from build123d import *

# Parameters (mm, degrees)
CROQUIS1_R               = 1.55
CROQUIS1_R_2             = 4
SALIENTE_EXTRUIR10_DEPTH = 3
CROQUIS2_R               = 8
CROQUIS2_R_2             = 1.55
CORTAR_EXTRUIR1_DEPTH    = 3
CROQUIS3_OUTSIDE_W       = 98.706
CROQUIS3_OUTSIDE_H       = 99.406
CROQUIS3_OUTSIDE_R       = 4
CROQUIS3_OUTSIDE_R_2     = 8
CROQUIS3_OUTSIDE_R_3     = 1.55
CORTAR_EXTRUIR2_DEPTH    = 3
REDONDEO1_R              = 6
REDONDEO2_R              = 3


with BuildPart() as part:
    # Croquis1 → Saliente-Extruir10 (new body)
    with BuildSketch(Plane(origin=(0, 0, 0), x_dir=(1, 0, 0), z_dir=(0, 1, 0))):
        Polygon((0, 0), (0, 38.7), (10, 38.7), (10, 42), (0, 42), (0, 72), (69.3, 72), (75.3, 72), (75.3, 52), (75.3, 42), (69.3, 42), (69.3, 51.7), (66, 51.7), (66, 42), (50, 42), (50, 38.7), (69.3, 38.7), (69.3, 0), (69.3, -4), (0, -4), align=None)
        with Locations((30, 40.2)):
            Circle(CROQUIS1_R, mode=Mode.SUBTRACT)
        with Locations((67.8, 61.7)):
            Circle(CROQUIS1_R, mode=Mode.SUBTRACT)
        with Locations((12.5, 9.4)):
            Circle(CROQUIS1_R_2, mode=Mode.SUBTRACT)
    extrude(amount=SALIENTE_EXTRUIR10_DEPTH)

    # Croquis2 → Cortar-Extruir1 (cut)
    with BuildSketch(Plane(origin=(0, 3, 0), x_dir=(1, 0, 0), z_dir=(0, 1, 0))):
        with Locations((29.5, 9.7)):
            Circle(CROQUIS2_R)
        with Locations((12.5, 17.4)):
            Circle(CROQUIS2_R_2)
        with Locations((12.5, 1.4)):
            Circle(CROQUIS2_R_2)
    extrude(amount=-CORTAR_EXTRUIR1_DEPTH, mode=Mode.SUBTRACT)

    # Croquis3 outside → Cortar-Extruir2 (cut)
    with BuildSketch(Plane(origin=(0, 3, 0), x_dir=(1, 0, 0), z_dir=(0, 1, 0))):
        with Locations((37.65, 34)):
            Rectangle(CROQUIS3_OUTSIDE_W, CROQUIS3_OUTSIDE_H)
        with BuildLine():
            Line((75.3, 72), (63, 72))
            ThreePointArc((63, 72), (34.270978976, 52.034382388), (0, 45))
            Line((0, 45), (0, 42))
            Line((0, 42), (10, 42))
            Line((10, 42), (10, 38.7))
            Line((10, 38.7), (0, 38.7))
            Line((0, 38.7), (0, 9.7))
            ThreePointArc((0, 9.7), (5.916961411, -0.92608126), (18.066176471, -1.492304477))
            ThreePointArc((18.066176471, -1.492304477), (19.571107199, -2.84659666), (21.235013612, -4))
            Line((21.235013612, -4), (37.764986388, -4))
            ThreePointArc((37.764986388, -4), (43.432691452, 1.833608903), (45.5, 9.7))
            ThreePointArc((45.5, 9.7), (54.274410069, 25.678480622), (69.3, 36))
            Line((69.3, 36), (69.3, 38.7))
            Line((69.3, 38.7), (50, 38.7))
            Line((50, 38.7), (50, 42))
            Line((50, 42), (66, 42))
            Line((66, 42), (66, 51.7))
            Line((66, 51.7), (69.3, 51.7))
            Line((69.3, 51.7), (69.3, 42))
            Line((69.3, 42), (75.3, 42))
            Line((75.3, 42), (75.3, 72))
        make_face(mode=Mode.SUBTRACT)
        with Locations((12.5, 9.4)):
            Circle(CROQUIS3_OUTSIDE_R)
        with Locations((29.5, 9.7)):
            Circle(CROQUIS3_OUTSIDE_R_2)
        with Locations((30, 40.2)):
            Circle(CROQUIS3_OUTSIDE_R_3)
        with Locations((67.8, 61.7)):
            Circle(CROQUIS3_OUTSIDE_R_3)
    extrude(amount=-CORTAR_EXTRUIR2_DEPTH, mode=Mode.SUBTRACT)

    # Redondeo1
    redondeo1_edges = [part.edges().sort_by_distance(p)[0] for p in [
        (75.3, 1.5, -72),
    ]]
    fillet(redondeo1_edges, radius=REDONDEO1_R)

    # Redondeo2
    redondeo2_edges = [part.edges().sort_by_distance(p)[0] for p in [
        (0, 1.5, -45),
    ]]
    fillet(redondeo2_edges, radius=REDONDEO2_R)


solid = part.part
Source: CAD feature listing. Evaluate the final solid. Frame: model axes, mm. A direction names the side the tool comes from. Give positions to 0.01 mm unless a question says otherwise; leave off trailing zeros. Order: outer loops, then holes, each group sorted by start corner. A loop starts at its lowest first (then second) coordinate and runs counter-clockwise, first axis right, second up. Notation, with made-up numbers: (59, 86) -> (112, 86) arc R28 cw to (112, 119) -> close; hole circle Ø4 at (-3.75, 50). An arc over 180 degrees is marked (long way). Write item = value, one per line.
Item 1: Section query B-B (x = 29.5). Output: boundary loops of the cut face in (y, z), then the cut area to 3 significant figures.
Check result:
outline = (0, -50.15) -> (3, -50.15) -> (3, -41.67) -> (0, -41.67) -> close; (0, -38.73) -> (3, -38.73) -> (3, -17.7) -> (0, -17.7) -> close; (0, -1.7) -> (3, -1.7) -> (3, 4) -> (0, 4) -> close
area = 106 mm²
Item 2: Section query C-C (x = 15.5). Output: boundary loops of the cut face in (y, z), then the cut area to 3 significant figures.
Check result:
outline = (0, -46.39) -> (3, -46.39) -> (3, -12.05) -> (0, -12.05) -> close; (0, -6.75) -> (3, -6.75) -> (3, 2.43) -> (0, 2.43) -> close
area = 131 mm²
Item 3: Contact query for flat-ended pins moving along their axis: pin 1 (0.9 mm diameter, centred on x = 61.5, y = 2, fed in from +Z); pin 2 (1.5 mm diameter, centred on x = 40, y = 0.5, fed in from -Z); pin 3 (1.5 mm diameter, centred on y = 1, z = -40, fed in from +X). Output: stop coordinate, or through.
Check result:
pin_1 = -31.63
pin_2 = -55.13
pin_3 = 50
Item 4: Section query A-A (y = 1.2). State how many separate pieces and enclosed holes the cut face has, then the cut area to 3 significant figures.
Check result:
separate_pieces = 1
enclosed_holes = 6
area = 3,020 mm²
Item 5: Mould query, pull axis Z, two halves, no side actions, for faces 1 (the face through (19.55, 1.52, 2.83)), 2 (the face through (75.3, 1, -54)), 3 (the face through (60, 1, -38.7)). Classes: +Z half, -Z half, draft (parallel to the pull), parting line (faces both ways), or undercut.
Check result:
face_1 = +Z half
face_2 = draft
face_3 = undercut
Item 6: Set-up query: faces 4 (the face through (72, 1, -42)), 5 (the face through (5.766, 1.521, 0.831)), 6 (the face through (68, 1, -51.7)), 7 (the face through (58, 1, -42)), 8 (the face through (5, 1, -38.7)). Return all of +Z, -Z, +X, -X, +Y, -Y with unobstructed straight access to the full face (end or side cutting, diameter ignored); none if empty.
Check result:
face_4 = +Z, +X, +Y, -Y
face_5 = +Z, +Y, -Y
face_6 = +Y, -Y
face_7 = +X, +Y, -Y
face_8 = -X, +Y, -Y
Item 7: Ray query, probe 1 along X at (y, z) = (1.2, -9.4); probe 2 along Z at (x, y) = (12.5, 2.35); probe 3 along Z at (x, y) = (30, 1.4). Return the intervals inside material, ascending.
Check result:
probe_1 = 0 to 8.5, 16.5 to 21.51, 37.49 to 45.5
probe_2 = -45.9 to -18.95, -15.85 to -13.4, -5.4 to -2.95, 0.15 to 2.8
probe_3 = -50.34 to -41.75, -38.65 to -17.68, -1.72 to 4
Item 8: Section query D-D (z = -26). Output: boundary loops of the cut face in (x, y), then the cut area to 3 significant figures.
Check result:
outline = (0, 0) -> (54.57, 0) -> (54.57, 3) -> (0, 3) -> close
area = 164 mm²
